Work out the finished part from the listing and answer in its coordinate system (mm). Face numbers are marked on the shaded views. Coordinates: 2 decimals unless noted, no trailing zeros. Order: outer loops, then holes, each group sorted by start corner. A loop starts at its lowest first (then second) coordinate and runs counter-clockwise, first axis right, second up. Notation, with made-up numbers: (-7.75, 70) -> (33.25, 70) arc R18 cw to (33.25, 75) -> close; hole circle Ø8 at (57.5, 52). An arc over 180 degrees is marked (long way). Write item = value, one per line. Start each with the question number.
Q1. The part is cut by section B-B, the plane x = 25. Determine the outline of the cut face in (y, z), plus the area to 3 significant figures.
Q2. The part is cut by section D-D, the plane y = 31.5. Determine the outline of the cut face in (x, z).
Q3. Flat-ended cylindrical pins translate along their axes: pin 1 (6.5 mm diameter, centred on y = 26.5, z = 32.5, fed in from -X); pin 2 (6.5 mm diameter, centred on x = 37, z = 32.5, fed in from +Y); pin 3 (6.5 mm diameter, centred on y = 14.5, z = 34, fed in from -X). Find the tip coordinate at first contact, or state that the pin passes through.
Q4. For a pull along X with two mould halves and no side action, classify the marked faces 1, 2 and 3 as +X half, -X half, draft (parallel to the pull), parting line (faces both ways), or undercut.
Q5. The part is cut by section A-A, the plane y = 46. Determine the outline of the cut face in (x, z).
Q6. The part is cut by section C-C, the plane y = 24. Determine the outline of the cut face in (x, z).
Q7. Straight lines are drawn through the part: L1, parallel to Z at x = 11, y = 46; L2, parallel to Y at x = 16, z = 36. For each, find the intervals that lie inside material, in ascending order. Write a range as from..to.
```python
from build123d import *

# Parameters (mm, degrees)
F0_W     = 50
F0_H     = 50
F1_DEPTH = 50
F2_R     = 5
F3_R     = 4.215568
F4_DEPTH = 5
F5_R     = 4.215568
F6_DEPTH = 5
F7_R     = 4.1557
F8_DEPTH = 5


with BuildPart() as f1:
    # F0 (on Top) → F1 (new body)
    with BuildSketch(Plane.XY):
        with Locations((25, 25)):
            Rectangle(F0_W, F0_H)
    extrude(amount=F1_DEPTH)

    # F2
    f2_edges = [f1.edges().sort_by_distance(p)[0] for p in [
        (25, 0, 50),
        (50, 0, 25),
        (25, 0, 0),
        (0, 0, 25),
        (0, 25, 50),
        (0, 50, 25),
        (0, 25, 0),
        (25, 50, 50),
        (50, 25, 50),
        (50, 50, 25),
        (25, 50, 0),
        (50, 25, 0),
    ]]
    fillet(f2_edges, radius=F2_R)

    # F3 (on face) → F4 (cut)
    with BuildSketch(Plane.XZ):
        with Locations((13.303663, 33.014465)):
            Circle(F3_R)
        with Locations((24.503663, 33.014465)):
            Circle(F3_R)
        with Locations((35.703663, 33.014465)):
            Circle(F3_R)
        with Locations((13.440982, 16.774133)):
            Circle(F3_R)
        with Locations((24.640982, 16.774133)):
            Circle(F3_R)
        with Locations((35.840982, 16.774133)):
            Circle(F3_R)
    extrude(amount=-F4_DEPTH, mode=Mode.SUBTRACT)

    # F5 (on face) → F6 (cut)
    with BuildSketch(Plane(origin=(0, 0, 0), x_dir=(0, -1, 0), z_dir=(-1, 0, 0))):
        with Locations((-36.712744, 33.377577)):
            Circle(F5_R)
        with Locations((-25.512744, 33.377577)):
            Circle(F5_R)
        with Locations((-14.312744, 33.377577)):
            Circle(F5_R)
        with Locations((-32.08404, 17.225714)):
            Circle(F5_R)
        with Locations((-19.062114, 17.338414)):
            Circle(F5_R)
    extrude(amount=-F6_DEPTH, mode=Mode.SUBTRACT)

    # F7 (on face) → F8 (cut)
    with BuildSketch(Plane(origin=(0, 50, 0), x_dir=(-1, 0, 0), z_dir=(0, 1, 0))):
        with Locations((-12.061181, 16.614642)):
            Circle(F7_R)
        with Locations((-37.061181, 16.614642)):
            Circle(F7_R)
        with Locations((-12.061181, 33.114642)):
            Circle(F7_R)
        with Locations((-37.061181, 33.114642)):
            Circle(F7_R)
    extrude(amount=-F8_DEPTH, mode=Mode.SUBTRACT)


solid = f1.part
```
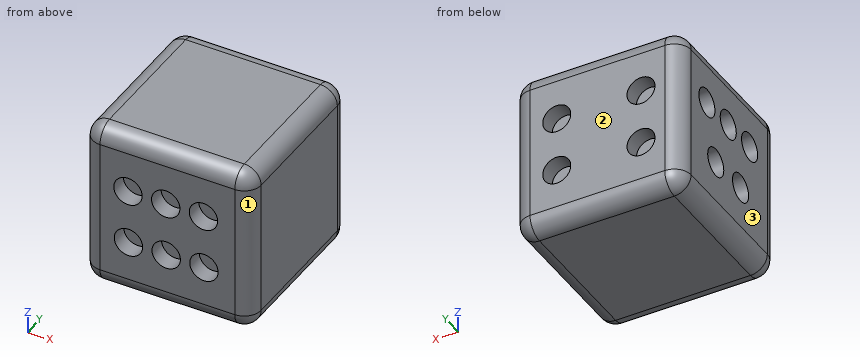
Model answer:
q1.outline = (0, 5) arc R5 ccw to (5, 0) -> (45, 0) arc R5 ccw to (50, 5) -> (50, 45) arc R5 ccw to (45, 50) -> (5, 50) arc R5 ccw to (0, 45) -> (0, 37.2) -> (5, 37.2) -> (5, 28.83) -> (0, 28.83) -> (0, 20.97) -> (5, 20.97) -> (5, 12.57) -> (0, 12.57) -> close
q1.area = 2,390 mm2
q2.outline = (0, 5) arc R5 ccw to (5, 0) -> (45, 0) arc R5 ccw to (50, 5) -> (50, 45) arc R5 ccw to (45, 50) -> (5, 50) arc R5 ccw to (0, 45) -> (0, 21.4) -> (5, 21.4) -> (5, 13.05) -> (0, 13.05) -> close
q3.pin_1 = 0
q3.pin_2 = 45
q3.pin_3 = 5
q4.face_1 = +X half
q4.face_2 = draft
q4.face_3 = -X half
q5.outline = (0.1, 5) arc R4.9 ccw to (5, 0.1) -> (45, 0.1) arc R4.9 ccw to (49.9, 5) -> (49.9, 45) arc R4.9 ccw to (45, 49.9) -> (5, 49.9) arc R4.9 ccw to (0.1, 45) -> close; hole circle Ø8.31 at (12.06, 16.61); hole circle Ø8.31 at (12.06, 33.11); hole circle Ø8.31 at (37.06, 16.61); hole circle Ø8.31 at (37.06, 33.11)
q6.outline = (0, 5) arc R5 ccw to (5, 0) -> (45, 0) arc R5 ccw to (50, 5) -> (50, 45) arc R5 ccw to (45, 50) -> (5, 50) arc R5 ccw to (0, 45) -> (0, 37.31) -> (5, 37.31) -> (5, 29.44) -> (0, 29.44) -> close
q7.L1 = 0.1..12.6, 20.63..29.1, 37.13..49.9
q7.L2 = 5..50
